Geometry check sheet. Reference: the model listing, model coordinates, mm. Face numbers are marked on the shaded views. A direction names the side the tool comes from. Round coordinates to 2 decimals unless told otherwise and drop trailing zeros. Write each loop counter-clockwise with the first axis right and the second up, starting at its lowest first coordinate (ties: lowest second). Pieces come first, ordered by that corner, then holes. Notation, with made-up numbers: M 85.25,35 L 104.25,35 A27 ccw 104.25,70 Z; hole C 5,10 d2. An arc over 180 degrees is marked long. Use a Markdown table: item, result.
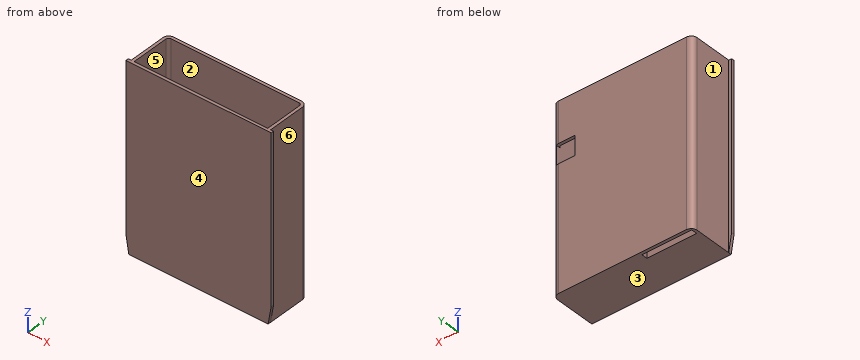
```python
from build123d import *

# Parameters (mm, degrees)
SKETCH1_W           = 72
SKETCH1_H           = 24
BOSS_EXTRUDE1_DEPTH = 95
SKETCH2_W           = 69
SKETCH2_H           = 21
CUT_EXTRUDE1_DEPTH  = 93
SKETCH3_W           = 10
SKETCH3_H           = 10
CUT_EXTRUDE2_DEPTH  = 2
SKETCH4_W           = 27.74
SKETCH4_H           = 5
BOSS_EXTRUDE2_DEPTH = 14
SKETCH5_W           = 25.74
SKETCH5_H           = 3
CUT_EXTRUDE3_DEPTH  = 16
SKETCH6_W           = 1.5
SKETCH6_H           = 1.5
BOSS_EXTRUDE4_DEPTH = 95
FILLET1_R           = 3
BOSS_EXTRUDE5_DEPTH = 1
FILLET2_R           = 1.5
CUT_EXTRUDE4_DEPTH  = 1.5


with BuildPart() as part:
    # Sketch1 → Boss-Extrude1 (new body)
    with BuildSketch(Plane.XY):
        with Locations((36, 12)):
            Rectangle(SKETCH1_W, SKETCH1_H)
    extrude(amount=BOSS_EXTRUDE1_DEPTH)

    # Sketch2 → Cut-Extrude1 (cut)
    with BuildSketch(Plane.XY.offset(95)):
        with Locations((36, 12)):
            Rectangle(SKETCH2_W, SKETCH2_H)
    extrude(amount=-CUT_EXTRUDE1_DEPTH, mode=Mode.SUBTRACT)

    # Sketch3 → Cut-Extrude2 (cut)
    with BuildSketch(Plane(origin=(0, 24, 0), x_dir=(1, 0, 0), z_dir=(0, 1, 0))):
        with Locations((65.5, -69)):
            Rectangle(SKETCH3_W, SKETCH3_H)
    extrude(amount=-CUT_EXTRUDE2_DEPTH, mode=Mode.SUBTRACT)

    # Sketch4 → Boss-Extrude2 (add)
    with BuildSketch(Plane.XY.offset(2)):
        with Locations((15.37, 20)):
            Rectangle(SKETCH4_W, SKETCH4_H)
    extrude(amount=BOSS_EXTRUDE2_DEPTH)

    # Sketch5 → Cut-Extrude3 (cut)
    with BuildSketch(Plane(origin=(0, 0, 0), x_dir=(-1, 0, 0), z_dir=(0, 0, -1))):
        with Locations((-14.37, 21)):
            Rectangle(SKETCH5_W, SKETCH5_H)
    extrude(amount=-CUT_EXTRUDE3_DEPTH, mode=Mode.SUBTRACT)

    # Sketch6 → Boss-Extrude4 (add)
    with BuildSketch(Plane(origin=(0, 0, 0), x_dir=(-1, 0, 0), z_dir=(0, 0, -1))):
        with Locations((-72.75, 0.75)):
            Rectangle(SKETCH6_W, SKETCH6_H)
        with Locations((0.75, 0.75)):
            Rectangle(SKETCH6_W, SKETCH6_H)
    extrude(amount=-BOSS_EXTRUDE4_DEPTH)

    # Fillet1
    # the kernel refuses this fillet: 3 mm, written as the material it takes off along each edge
    with BuildSketch(Plane(origin=(0, 24, -7.5), x_dir=(1, 0, 0), z_dir=(0, 0, 1)), Plane(origin=(72, 24, -7.5), x_dir=(0, -1, 0), z_dir=(0, 0, 1))) as fillet1_piece_1:
        with BuildLine():
            CenterArc((FILLET1_R, -FILLET1_R), FILLET1_R, 90, 90)
            Line((0, -FILLET1_R), (0, 0))
            Line((0, 0), (FILLET1_R, 0))
        make_face()
    extrude(amount=110, mode=Mode.SUBTRACT)

    # Sketch7 → Boss-Extrude5 (add)
    with BuildSketch(Plane.XY.offset(16)):
        Polygon((29.24, 22.5), (26.24, 22.5), (26.24, 19.5), (3.1, 19.5), (3.1, 22.5), (1.5, 22.5), (1.5, 17.5), (3.1, 17.5), (26.24, 17.5), (29.24, 17.5), align=None)
    extrude(amount=BOSS_EXTRUDE5_DEPTH)

    # Fillet2
    fillet2_edges = [part.edges().sort_by_distance(p)[0] for p in [
        (1.5, 22.5, 56),
        (70.5, 22.5, 33),
        (70.5, 22.5, 84.5),
    ]]
    fillet(fillet2_edges, radius=FILLET2_R)

    # Sketch8 → Cut-Extrude4 (cut)
    with BuildSketch(Plane(origin=(0, 0, 0), x_dir=(-1, 0, 0), z_dir=(0, -1, 0))):
        Polygon((0, 0), (1.5, -9.268975532), (1.5, 0), align=None)
        Polygon((-73.5, -9.268975532), (-71.934797197, 0), (-73.5, 0), align=None)
    extrude(amount=-CUT_EXTRUDE4_DEPTH, mode=Mode.SUBTRACT)


solid = part.part
```
Item 1: Cross-section at A-A, the plane x = 18.5. Record the cut outline in (y, z).
Outcome:
| item | result |
|---|---|
| outline | M 0,0 L 19.5,0 L 19.5,17 L 17.5,17 L 17.5,2 L 1.5,2 L 1.5,95 L 0,95 Z; M 22.5,0 L 24,0 L 24,95 L 22.5,95 Z |
Item 2: Material ranges on line 1 along X through (y, z) = (21, 6.5); line 2 along X through (y, z) = (6, 31); line 3 along Y through (x, z) = (30, 87.5), recorded low to high. Write a range as from..to.
Outcome:
| item | result |
|---|---|
| line 1 | x = 0..1.5, 27.24..29.24, 70.5..72 |
| line 2 | x = 0..1.5, 70.5..72 |
| line 3 | y = 0..1.5, 22.5..24 |
Item 3: Cross-section at D-D, the plane x = 56.5. Record the cut outline in (y, z), and give its area (3 significant figures).
Outcome:
| item | result |
|---|---|
| outline | M 0,0 L 24,0 L 24,95 L 22.5,95 L 22.5,2 L 1.5,2 L 1.5,95 L 0,95 Z |
| area | 327 mm2 |
Item 4: Mould release check, pull along X, two halves, no side actions. Record for the marked faces 1, 2 and 3: +X half, -X half, draft (parallel to the pull), parting line (faces both ways), or undercut.
Outcome:
| item | result |
|---|---|
| face 1 | -X half |
| face 2 | undercut |
| face 3 | draft |
Item 5: Cross-section at B-B, the plane z = 55.5. Record the cut outline in (x, y), and give its area (3 significant figures).
Outcome:
| item | result |
|---|---|
| outline | M -1.5,0 L 73.5,0 L 73.5,1.5 L 72,1.5 L 72,21 A3 ccw 69,24 L 3,24 A3 ccw 0,21 L 0,1.5 L -1.5,1.5 Z; hole M 1.5,1.5 L 70.5,1.5 L 70.5,21 A1.5 ccw 69,22.5 L 3,22.5 A1.5 ccw 1.5,21 Z |
| area | 281 mm2 |
Item 6: Access from +Z, -Z, +X, -X, +Y, -Y to the whole of each face (thin tool, end or side, straight path). Record for the marked faces 4, 5 and 6.
Outcome:
| item | result |
|---|---|
| face 4 | +Z, -Z, +X, -X, -Y |
| face 5 | +Z |
| face 6 | +Z, -Z, +X, +Y |
Item 7: Go/stop test with flat-tipped pins: pin 1 (0.5 mm diameter, centred on y = 21, z = 16.5, fed in from +X); pin 2 (1.5 mm diameter, centred on y = 21.5, z = 6, fed in from -X); pin 3 (1.5 mm diameter, centred on x = 14, z = 16, fed in from -Y); pin 4 (6.5 mm diameter, centred on x = 35, y = 11.5, fed in from +Z). Record where each tip stops, or that it passes through.
Outcome:
| item | result |
|---|---|
| pin 1 | stops at x = 72 |
| pin 2 | stops at x = 0 |
| pin 3 | stops at y = 0 |
| pin 4 | stops at z = 2 |
Item 8: Cross-section at C-C, the plane y = 7.25. Record the cut outline in (x, z), and give its area (3 significant figures).
Outcome:
| item | result |
|---|---|
| outline | M 0,0 L 72,0 L 72,95 L 70.5,95 L 70.5,2 L 1.5,2 L 1.5,95 L 0,95 Z |
| area | 423 mm2 |
